Part model, mm, in its own coordinate system. Face numbers are marked on the shaded views. A direction names the side the tool comes from. Give positions to 0.01 mm unless a question says otherwise; leave off trailing zeros. Write each loop counter-clockwise with the first axis right and the second up, starting at its lowest first coordinate (ties: lowest second). Pieces come first, ordered by that corner, then holes.
Autodesk Inventor part; units mm, degrees
ref_plane "YZ Plane" through (0, 0, 0) normal (1, 0, 0) x (0, 1, 0)
ref_plane "XZ Plane" through (0, 0, 0) normal (0, 1, 0) x (-1, 0, 0)
ref_plane "XY Plane" through (0, 0, 0) normal (0, 0, 1) x (1, 0, 0)
sketch "Sketch1" plane through (0, 0, 0) normal (1, 0, 0) x (0, 1, 0)
  line L0 (0, 0) -> (0, 597.7382)
  line L1 (0, 0) -> (3.175, 0)
  line L2 (3.175, 0) -> (3.175, 594.5632)
  line L3 (3.175, 594.5632) -> (9.906, 594.5632)
  line L4 (9.906, 594.5632) -> (15.756, 595.9828)
  line L5 (0, 597.7382) -> (9.5263, 597.7382)
  line L6 (9.5263, 597.7382) -> (12.7824, 598.5283)
  line L7 (41.2921, 902.0052) -> (15.756, 595.9828)
  line L8 (12.7824, 598.5283) -> (38.1281, 902.2692)
  line L9 (38.1281, 902.2692) -> (41.2921, 902.0052)
  line L10 (41.2921, 902.0052) -> (44.4671, 901.7403)
  line L11 (44.4671, 901.7403) -> (18.7409, 593.44)
  line L12 (18.7409, 593.44) -> (10.2857, 591.3882)
  line L13 (10.2857, 591.3882) -> (6.35, 591.3882)
  line L14 (6.35, 591.3882) -> (6.35, 574.5988)
  line L15 (6.35, 574.5988) -> (3.175, 574.5988)
  line L16 (44.4671, 901.7403) -> (47.6311, 901.4763)
  line L17 (47.6311, 901.4763) -> (21.7146, 590.8944)
  line L18 (21.7146, 590.8944) -> (10.6654, 588.2132)
  line L19 (10.6654, 588.2132) -> (9.525, 588.2132)
  line L20 (9.525, 588.2132) -> (9.525, 432.9684)
  line L21 (9.525, 432.9684) -> (6.35, 432.9684)
  line L22 (6.35, 432.9684) -> (6.35, 574.5988)
  line L23 (32.5862, 759.3601) -> (35.7502, 759.0961)
  point P0 (14.5133, 592.4141)
  dimension "d0" = 594.5632
  dimension "d1" = 3.175
  dimension "d2" = 6.731
  dimension "d7" = 3.175
  dimension "d8" = 6.0198
  dimension "d9" = 166.36
  dimension "d10" = 3.175
  dimension "d11" = 108.41
  dimension "d12" = 3.175
  dimension "d13" = 307.086
  dimension "d18" = 3.175
  dimension "d20" = 307.1025
  dimension "d21" = 8.7006
  dimension "d22" = 3.175
  dimension "d23" = 3.175
  dimension "d24" = 3.9357
  dimension "d25" = 16.7894
  dimension "d28" = 3.175
  dimension "d29" = 3.186
  dimension "d30" = 3.175
  dimension "d32" = 3.175
  dimension "d33" = 3.175
  dimension "d34" = 142.875
  dimension "d35" = 168.7862
  dimension "d36" = 11.3698
  dimension "d37" = 1.1404
  dimension "d38" = 155.2448
extrude "Extrusion3" add sketch "Sketch1" along normal blind 1000.125 contours L14 L13 L12 L11 L23 L17 L18 L19 L20 L21 L22
properties part number "Second_Shingle_Over_Intake_Vent_With_Length_39.375_Inches"
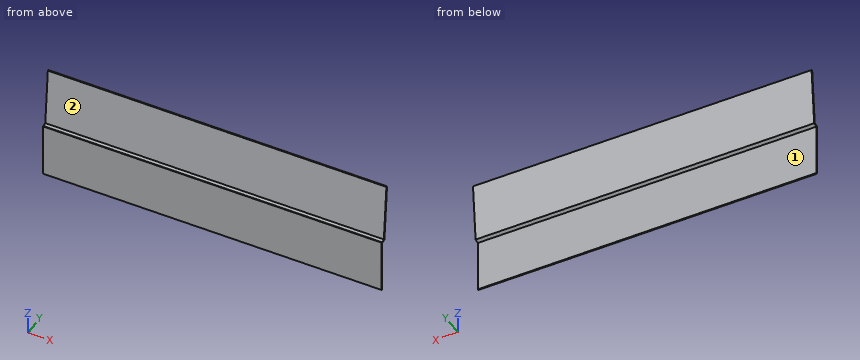
1) Flat gauge pins, fed straight in: P1, Ø6, axis at x = 315, z = 677.5, coming from the +Y side; P2, Ø8, axis at x = 690.5, z = 487.5, coming from the +Y side (3 decimals); P3, Ø2, axis at x = 389, z = 616, coming from the +Y side; P4, Ø6, axis at y = 14.5, z = 564.5, coming from the -X side. Where does each tip first touch, or does it go through?
Check result:
P1: stops at y = 29.19
P2: stops at y = 9.525
P3: stops at y = 23.89
P4: passes through
2) Saw through at B-B (z = 488.5). Write the cut outline in (x, y) (3 decimals).
Check result:
outline: (0, 6.35) - (1000.125, 6.35) - (1000.125, 9.525) - (0, 9.525) - close
3) 3-axis set-ups, long thin cutter, end or side, ignore diameter. For the marked faces 1 and 2: which of +Z, -Z, +X, -X, +Y, -Y reach the whole face in a straight line?
Check result:
face 1: -Z, +X, -X, +Y
face 2: +Z, +X, -X, -Y
4) Drill centre lines: L1, parallel to Y at x = 502.5, z = 493 (3 decimals); L2, parallel to Y at x = 413, z = 690; L3, parallel to Z at x = 211, y = 15. Where is each one in solid material? Low to high.
Check result:
L1: y = 6.35 to 9.525
L2: y = 26.8 to 29.98
L3: z = 589.27 to 592.53
5) Saw through at C-C (z = 697). Write the cut outline in (x, y) (1 decimal).
Check result:
outline: (0, 27.4) - (1000.1, 27.4) - (1000.1, 30.6) - (0, 30.6) - close
6) Saw through at A-A (x = 668.5). Write the cut outline in (y, z) (3 decimals).
Check result:
outline: (6.35, 432.968) - (9.525, 432.968) - (9.525, 588.213) - (10.665, 588.213) - (21.715, 590.894) - (35.75, 759.096) - (32.586, 759.36) - (18.741, 593.44) - (10.286, 591.388) - (6.35, 591.388) - close
